Geometry: final body of the model. Coordinates: model frame, mm. A direction names the side the tool comes from. Round coordinates to 2 decimals unless told otherwise and drop trailing zeros. Write each loop counter-clockwise with the first axis right and the second up, starting at its lowest first coordinate (ties: lowest second). Pieces come first, ordered by that corner, then holes. Notation, with made-up numbers: M 56.25,6 L 97.25,6 A25 cw 97.25,22 Z; hole C 11,75 d6. An arc over 180 degrees is marked long. Use one line per item in the form item = value. Start each with the question number.
Item 1: Section query A-A (z = -12.5). Return loops of the section in (x, y).
Item 2: Section query C-C (x = -80). Return loops of the section in (y, z), and give its area (3 significant figures).
Item 3: Reachability of faces 1 (the flat face through (-15, 11, 0)), 2 (the flat face through (-46, 10, -31.5)), 3 (the cylindrical face through (-100.494, 2.465, -29.501)), 4 (the cylindrical face through (-14.79, 12.89, -43.66)), 5 (the flat face through (-15, 3.137, -30)) from +Z, -Z, +X, -X, +Y, -Y: full face, straight path, thin tool, end or side. Return the list, or none.
Item 4: Pin query (flat end, axial travel): pin 1 Ø6 at (x, z) = (-50.5, -10) entering from +Y; pin 2 Ø5 at (y, z) = (8.5, -44) entering from +X; pin 3 Ø2 at (x, y) = (-81.5, 3.5) entering from -Z; pin 4 Ø4 at (x, z) = (-92.9, -42.9) entering from -Y. Return the tip coordinate at first contact, or that it passes through.
Item 5: Section query D-D (y = 11.25). Return loops of the section in (x, z).
Item 6: Ray query, probe 1 along Z at (x, y) = (-63, 14.25); probe 2 along Z at (x, y) = (-70, 13.5); probe 3 along X at (y, z) = (13.25, -26.5). Return the intervals inside material, ascending.
Item 7: Section query B-B (x = -42.5). Return loops of the section in (y, z), and give its area (3 significant figures).
Item 8: Pull-direction query (X, two-part tool) for faces 6 (the flat face through (-15, 5.9, -4)), 7 (the cylindrical face through (-64.136, 9.93, -27.917)), 8 (the flat face through (-56.99, 7.89, -3.92)); classes: pulls with the +X half, pulls with the -X half, needs draft (parallel to the pull), parting line crosses it, or undercut.
from build123d import *

# Parameters (mm, degrees)
EXTRUDE_1_DEPTH      = 16
SKETCH_2_R           = 16
CUT_EXTRUDE_1_DEPTH  = 15
SKETCH_3_R           = 13
CUT_EXTRUDE_2_DEPTH  = 120.713198938
SKETCH_4_R           = 20.5
CUT_EXTRUDE_3_DEPTH  = 5
HOLE_WIZARD_M32_D    = 3.4
CUT_EXTRUDE_8_DEPTH  = 30
CUT_EXTRUDE_11_DEPTH = 120.842605112
EXTRUDE_2_DEPTH      = 11


with BuildPart() as part:
    # Эскиз1 → Бобышка-Вытянуть1 (new body)
    with BuildSketch(Plane(origin=(0, 0, 0), x_dir=(1, 0, 0), z_dir=(0, 1, 0))):
        with BuildLine():
            Line((0, 0), (0, 60))
            Line((0, 60), (-30, 60))
            Line((-30, 60), (-83.234756238, 52.266260397))
            ThreePointArc((-83.234756238, 52.266260397), (-102.5, 30), (-83.234756238, 7.733739603))
            Line((-83.234756238, 7.733739603), (-30, 0))
            Line((-30, 0), (0, 0))
        make_face()
    extrude(amount=EXTRUDE_1_DEPTH)

    # Эскиз2 → Вырез-Вытянуть1 (cut)
    with BuildSketch(Plane.XZ):
        with Locations(Location((-80, -30, 0), (0, 0, 270))):
            Circle(SKETCH_2_R)
    extrude(amount=-CUT_EXTRUDE_1_DEPTH, mode=Mode.SUBTRACT)

    # Эскиз3 → Вырез-Вытянуть2 (cut, through all)
    with BuildSketch(Plane.XZ.offset(-15)):
        with Locations(Location((-80, -30, 0), (0, 0, 270))):
            Circle(SKETCH_3_R)
    extrude(amount=-CUT_EXTRUDE_2_DEPTH, mode=Mode.SUBTRACT)

    # Эскиз4 → Вырез-Вытянуть3 (cut)
    with BuildSketch(Plane.XZ):
        with Locations(Location((-80, -30, 0), (0, 0, 270))):
            Circle(SKETCH_4_R)
    extrude(amount=-CUT_EXTRUDE_3_DEPTH, mode=Mode.SUBTRACT)

    # Отверстие с зазором M32 (through all)
    with Locations(Plane(origin=(0, 5, 0), x_dir=(-1, 0, 0), z_dir=(0, -1, 0))):
        with Locations((92.904698757, 17.095301243), (67.095301243, 17.095301243), (67.095301243, 42.904698757), (92.904698757, 42.904698757)):
            Hole(HOLE_WIZARD_M32_D / 2)

    # Эскиз8 → Вырез-Вытянуть8 (cut)
    with BuildSketch(Plane(origin=(0, 0, 0), x_dir=(0, 0, -1), z_dir=(1, 0, 0))):
        with BuildLine():
            Line((38.359861864, 3.136561351), (21.640138136, 3.136561351))
            ThreePointArc((21.640138136, 3.136561351), (16.509790629, 12.858627047), (8, 5.9))
            Line((8, 5.9), (0, 5.9))
            Line((0, 5.9), (0, 0))
            Line((0, 0), (60, 0))
            Line((60, 0), (60, 5.9))
            Line((60, 5.9), (52, 5.9))
            ThreePointArc((52, 5.9), (43.490209371, 12.858627047), (38.359861864, 3.136561351))
        make_face()
    extrude(amount=-CUT_EXTRUDE_8_DEPTH, mode=Mode.SUBTRACT)

    # Эскиз14 → Вырез-Вытянуть11 (cut, through all)
    with BuildSketch(Plane.XZ):
        with BuildLine():
            Line((-33, -56.53267916), (-76.544602266, -50.206687668))
            ThreePointArc((-76.544602266, -50.206687668), (-59.5, -30), (-76.544602266, -9.793312332))
            Line((-76.544602266, -9.793312332), (-33, -3.46732084))
            Line((-33, -3.46732084), (-33, -56.53267916))
        make_face()
    extrude(amount=-CUT_EXTRUDE_11_DEPTH, mode=Mode.SUBTRACT)

    # Эскиз15 → Бобышка-Вытянуть2 (add, through all)
    with BuildSketch(Plane.XZ.offset(-5)):
        with BuildLine():
            Line((-59.5549517, -31.5), (-33, -31.5))
            Line((-33, -31.5), (-33, -28.5))
            Line((-33, -28.5), (-59.5549517, -28.5))
            ThreePointArc((-59.5549517, -28.5), (-59.5, -30), (-59.5549517, -31.5))
        make_face()
    extrude(amount=-EXTRUDE_2_DEPTH)


solid = part.part
Working result:
q1.outline = M -94.14,0 L -90.68,0 L -90.68,5 L -69.32,5 L -69.32,16 L -94.14,16 Z; M -33,0 L -30,0 L -30,12.51 L 0,12.51 L 0,16 L -33,16 Z
q2.outline = M 0,-52.74 L 16,-52.74 L 16,-43 L 15,-43 L 15,-46 L 5,-46 L 5,-50.5 L 0,-50.5 Z; M 0,-9.5 L 5,-9.5 L 5,-14 L 15,-14 L 15,-17 L 16,-17 L 16,-7.26 L 0,-7.26 Z
q2.area = 177 mm²
q3.face_1 = +Z, +X, -X, +Y, -Y
q3.face_2 = +Y, -Y
q3.face_3 = -Y
q3.face_4 = +X
q3.face_5 = +Z, -Z, +X, -Y
q4.pin_1 = through
q4.pin_2 = -30
q4.pin_3 = -52.66
q4.pin_4 = 5
q5.outline = M -83.23,-52.27 L -30,-60 L 0,-60 L 0,-49.57 L -30,-49.57 L -30,-40.23 L 0,-40.23 L 0,-19.77 L -30,-19.77 L -30,-10.43 L 0,-10.43 L 0,0 L -30,0 L -83.23,-7.73 A22.5 ccw Z; hole C -80,-30 d32; hole C -92.9,-42.9 d3.4; hole C -92.9,-17.1 d3.4; hole M -76.54,-50.21 L -33,-56.53 L -33,-31.5 L -59.55,-31.5 A20.5 cw Z; hole M -76.54,-9.79 A20.5 cw -59.55,-28.5 L -33,-28.5 L -33,-3.47 Z; hole C -67.1,-42.9 d3.4; hole C -67.1,-17.1 d3.4
q6.probe_1 = -55.21 to -52.17, -41.46 to -18.54, -7.83 to -4.79
q6.probe_2 = -54.19 to -51.16, -47.9 to -42.49, -17.51 to -12.1, -8.84 to -5.81
q6.probe_3 = -102.23 to -95.61, -64.39 to -59.8, -33 to 0
q7.outline = M 0,-58.18 L 16,-58.18 L 16,-55.15 L 0,-55.15 Z; M 0,-4.85 L 16,-4.85 L 16,-1.82 L 0,-1.82 Z; M 5,-31.5 L 16,-31.5 L 16,-28.5 L 5,-28.5 Z
q7.area = 130 mm²
q8.face_6 = needs draft
q8.face_7 = undercut
q8.face_8 = pulls with the -X half
